The model under review builds one solid part; all positions refer to its coordinate system, in mm. Coordinates: 2 decimals unless noted, no trailing zeros. Order: outer loops, then holes, each group sorted by start corner. A loop starts at its lowest first (then second) coordinate and runs counter-clockwise, first axis right, second up.
```python
from build123d import *

# Parameters (mm, degrees)
SKETCH1_R           = 85.725
BOSS_EXTRUDE1_DEPTH = 114.3
CUT_EXTRUDE1_DEPTH  = 152.4
SKETCH3_R           = 2.778125
CUT_EXTRUDE2_DEPTH  = 12.7
SKETCH4_R           = 6.985
CUT_EXTRUDE3_DEPTH  = 6.096


with BuildPart() as part:
    # Sketch1 → Boss-Extrude1 (new body)
    with BuildSketch(Plane(origin=(0, 0, 0), x_dir=(1, 0, 0), z_dir=(0, 1, 0))):
        Circle(SKETCH1_R)
    extrude(amount=BOSS_EXTRUDE1_DEPTH)

    # Sketch2 → Cut-Extrude1 (cut)
    with BuildSketch(Plane(origin=(0, 114.3, 0), x_dir=(1, 0, 0), z_dir=(0, 1, 0))):
        Polygon((85.724933621, -0.10668), (0, -85.725), (-45.627504124, -96.719379999), (-137.428949547, 46.173941299), (19.12530113, 101.910533163), (109.833872203, 30.600481808), align=None)
    extrude(amount=-CUT_EXTRUDE1_DEPTH, mode=Mode.SUBTRACT)

    # Sketch3 → Cut-Extrude2 (cut)
    with BuildSketch(Plane(origin=(42.862466811, 0, 42.91584), x_dir=(-0.707546622, 0, 0.706666667), z_dir=(-0.706666667, 0, -0.707546622))):
        with Locations((-37.719, 87.122)):
            Circle(SKETCH3_R)
        with Locations((-14.859, 87.122)):
            Circle(SKETCH3_R)
        with Locations((-37.719, 29.21)):
            Circle(SKETCH3_R)
        with Locations((-14.859, 29.21)):
            Circle(SKETCH3_R)
    extrude(amount=-CUT_EXTRUDE2_DEPTH, mode=Mode.SUBTRACT)

    # Sketch4 → Cut-Extrude3 (cut)
    with BuildSketch(Plane(origin=(0, 0, 0), x_dir=(-1, 0, 0), z_dir=(0, -1, 0))):
        with Locations((-51.720733405, -51.785137083)):
            Circle(SKETCH4_R)
    extrude(amount=-CUT_EXTRUDE3_DEPTH, mode=Mode.SUBTRACT)


solid = part.part
```
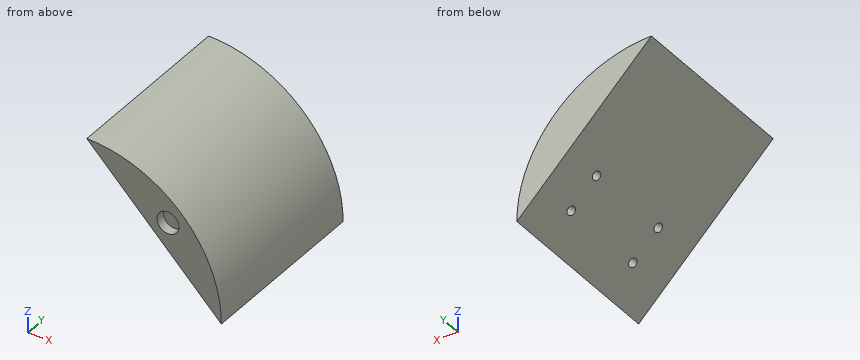
(1) We need section A-A, the plane x = 48. Write out the cut boundary in (y, z).
A:
outline: (0, 37.78) - (114.3, 37.78) - (114.3, 71.03) - (0, 71.03) - (0, 57.7) - (6.1, 57.7) - (6.1, 45.87) - (0, 45.87) - close
(2) For pin 1 Ø3 at (y, z) = (81, 65) entering from +X; pin 2 Ø8.5 at (x, z) = (51.72, 51.79) entering from -Y; pin 3 Ø1.5 at (x, y) = (38.5, 80.5) entering from -Z, all flat-tipped, find the tip position at first contact; note any pin that passes through.
A:
pin 1: stops at x = 57.59
pin 2: stops at y = 6.1
pin 3: stops at z = 46.52
(3) We need section D-D, the plane x = 19.5. Write out the cut boundary in (y, z).
A:
outline: (0, 66.25) - (114.3, 66.25) - (114.3, 83.48) - (0, 83.48) - close
(4) We need section B-B, the plane y = 57.5. Write out the cut boundary in (x, z) (3 decimals).
A:
outline: (0, 85.725) - (85.725, 0.107) arc R85.725 ccw to start
(5) We need section C-C, the plane z = 68. Write out the cut boundary in (x, y), and give its area (3 significant figures).
A:
outline: (17.75, 0) - (52.2, 0) - (52.2, 114.3) - (17.75, 114.3) - close
area: 3,940 mm2
(6) Wall thickness on probe 1 along X at (y, z) = (60, 71.5); probe 2 along Z at (x, y) = (23.5, 67); probe 3 along Z at (x, y) = (8.5, 88): over which ranges is each line inside the solid? List them lowest first.
A:
probe 1: x = 14.24 to 47.29
probe 2: z = 62.25 to 82.44
probe 3: z = 77.24 to 85.3
